from build123d import *

# Parameters (mm, degrees)
SALIENTE_EXTRUIR1_DEPTH = 3
CROQUIS2_W              = 65
CROQUIS2_H              = 19
SALIENTE_EXTRUIR2_DEPTH = 3
CROQUIS3_W              = 81.5
CROQUIS3_H              = 19
SALIENTE_EXTRUIR3_DEPTH = 3
CROQUIS4_R              = 1.5
CORTAR_EXTRUIR1_DEPTH   = 69
CROQUIS5_R              = 1.5
CORTAR_EXTRUIR2_DEPTH   = 82.5


with BuildPart() as part:
    # Croquis1 → Saliente-Extruir1 (new body)
    with BuildSketch(Plane(origin=(0, 0, 0), x_dir=(1, 0, 0), z_dir=(0, 1, 0))):
        Polygon((-39.25, -2.5), (14.25, -2.5), (14.25, -32.5), (39.25, -32.5), (39.25, 32.5), (-39.25, 32.5), align=None)
    extrude(amount=SALIENTE_EXTRUIR1_DEPTH)

    # Croquis2 → Saliente-Extruir2 (add)
    with BuildSketch(Plane(origin=(39.25, 0, 0), x_dir=(0, 0, -1), z_dir=(1, 0, 0))):
        with Locations((0, 9.5)):
            Rectangle(CROQUIS2_W, CROQUIS2_H)
    extrude(amount=SALIENTE_EXTRUIR2_DEPTH)

    # Croquis3 → Saliente-Extruir3 (add)
    with BuildSketch(Plane(origin=(0, 0, -32.5), x_dir=(-1, 0, 0), z_dir=(0, 0, -1))):
        with Locations((-1.5, 9.5)):
            Rectangle(CROQUIS3_W, CROQUIS3_H)
    extrude(amount=SALIENTE_EXTRUIR3_DEPTH)

    # Croquis4 → Cortar-Extruir1 (cut, through all)
    with BuildSketch(Plane(origin=(0, 0, -35.5), x_dir=(-1, 0, 0), z_dir=(0, 0, -1))):
        with Locations((31.75, 11.75)):
            Circle(CROQUIS4_R)
        with Locations((16.75, 11.75)):
            Circle(CROQUIS4_R)
    extrude(amount=-CORTAR_EXTRUIR1_DEPTH, mode=Mode.SUBTRACT)

    # Croquis5 → Cortar-Extruir2 (cut, through all)
    with BuildSketch(Plane(origin=(42.25, 0, 0), x_dir=(0, 0, -1), z_dir=(1, 0, 0))):
        with Locations((-25, 11.75)):
            Circle(CROQUIS5_R)
        with Locations((-10, 11.75)):
            Circle(CROQUIS5_R)
    extrude(amount=-CORTAR_EXTRUIR2_DEPTH, mode=Mode.SUBTRACT)


solid = part.part
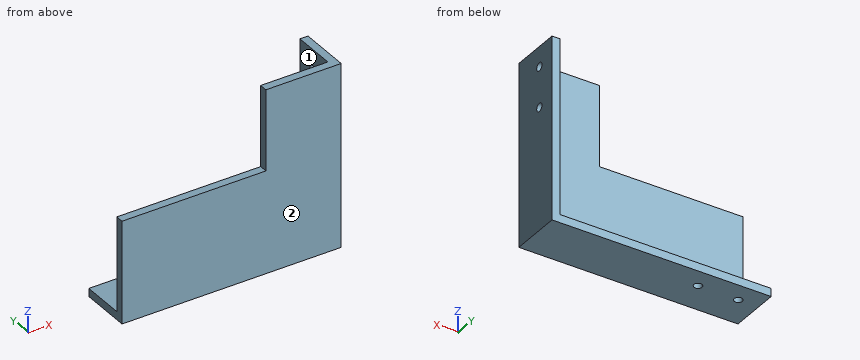
The listing builds one solid part. Answer for the finished solid, in the listing's coordinates (mm). Face numbers are marked on the shaded views. A direction names the side the tool comes from. Round coordinates to 2 decimals unless told otherwise and drop trailing zeros. Write each loop counter-clockwise with the first axis right and the second up, starting at its lowest first coordinate (ties: lowest second). Pieces come first, ordered by that corner, then holes. Notation, with made-up numbers: (-27.75, -22.5) - (8.25, -22.5) arc R20 cw to (8.25, 15.5) - close; hole circle Ø10 at (-4.75, 26.25). An arc over 180 degrees is marked (long way). Use a Markdown table: item, result. Add a question column.
1. A tool of negligible diameter and unlimited length cuts with its end or side. For the marked faces 1 and 2, from which of +Z, -Z, +X, -X, +Y, -Y can it reach the whole face along a straight path? Write none if from no direction.
2. The part is cut by section D-D (y = 4.25). Write down the section's boundary in (x, z).
3. The part is cut by section B-B (y = 11.75). Write down the section's boundary in (x, z), and give its area (4 significant figures).
4. The part is cut by section C-C (x = -31.75). Write down the section's boundary in (y, z).
5. The part is cut by section A-A (z = 10). Write down the section's boundary in (x, y).
6. Flat-ended cylindrical pins translate along their axes: P1, Ø1.5, axis at x = 12, y = 6.5, coming from the +Z side; P2, Ø3.5, axis at y = 1, z = 13.5, coming from the -X side; P3, Ø0.9, axis at x = -9, y = 1.5, coming from the +Z side. Find the tip coordinate at first contact, or state that the pin passes through.
7. Consider line 1 (Y direction, x = 41.4, z = 25); line 2 (Y direction, x = -9, z = -10); line 3 (Z direction, x = -25, y = 6.5). Determine where each line is inside the solid, lowest interval first.
Reported:
| question | item | result |
|---|---|---|
| 1 | face 1 | +Z, -X, +Y |
| 1 | face 2 | +Z, -Z, +X, -X, -Y |
| 2 | outline | (-39.25, -35.5) - (42.25, -35.5) - (42.25, 32.5) - (39.25, 32.5) - (39.25, -32.5) - (-39.25, -32.5) - close |
| 3 | outline | (-39.25, -35.5) - (-33.25, -35.5) - (-33.25, -32.5) - (-39.25, -32.5) - close; (-30.25, -35.5) - (-18.25, -35.5) - (-18.25, -32.5) - (-30.25, -32.5) - close; (-15.25, -35.5) - (42.25, -35.5) - (42.25, 8.5) - (39.25, 8.5) - (39.25, -32.5) - (-15.25, -32.5) - close; (39.25, 11.5) - (42.25, 11.5) - (42.25, 23.5) - (39.25, 23.5) - close; (39.25, 26.5) - (42.25, 26.5) - (42.25, 32.5) - (39.25, 32.5) - close |
| 3 | area | 403.5 mm^2 |
| 4 | outline | (0, -35.5) - (10.25, -35.5) - (10.25, -32.5) - (3, -32.5) - (3, 2.5) - (0, 2.5) - close; (13.25, -35.5) - (19, -35.5) - (19, -32.5) - (13.25, -32.5) - close |
| 5 | outline | (14.25, 0) - (42.25, 0) - (42.25, 10.25) - (39.25, 10.25) - (39.25, 3) - (14.25, 3) - close; (39.25, 13.25) - (42.25, 13.25) - (42.25, 19) - (39.25, 19) - close |
| 6 | P1 | z = -32.5 |
| 6 | P2 | x = 14.25 |
| 6 | P3 | z = 2.5 |
| 7 | line 1 | 0 to 10.25, 13.25 to 19 |
| 7 | line 2 | 0 to 3 |
| 7 | line 3 | -35.5 to -32.5 |
